```python
from build123d import *

# Parameters (mm, degrees)
F1_DEPTH = 10
F2_W     = 79.171128571
F2_H     = 17.1256698668
F3_DEPTH = 3
F6_R     = 24.75004298
F6_R_2   = 14.8028536267
F7_DEPTH = 3


# Not quite as in the source:
# - a fillet or chamfer that OpenCascade refuses, or shapes differently, is made with other operations: its cross-section is extruded or revolved along the edge and cut away or added


with BuildPart() as f1:
    # F0 (on Top) → F1 (new body)
    with BuildSketch(Plane.XY):
        with BuildLine():
            Line((-29.7593586147, -18.6613375429), (-29.7593586147, -52.9211238027))
            Line((-29.7593586147, -52.9211238027), (29.7593586147, -52.9211238027))
            Line((29.7593586147, -52.9211238027), (29.7593586147, -18.6613375429))
            ThreePointArc((29.7593586147, -18.6613375429), (0, -35.1264137658), (-29.7593586147, -18.6613375429))
        make_face()
        with BuildLine():
            ThreePointArc((-29.7593586147, 18.6613375429), (-35.1264137658, 0), (-29.7593586147, -18.6613375429))
            Line((-29.7593586147, -18.6613375429), (-29.7593586147, 18.6613375429))
        make_face()
        with BuildLine():
            Line((-29.7593586147, 18.6613375429), (-29.7593586147, -18.6613375429))
            ThreePointArc((-29.7593586147, -18.6613375429), (0, -35.1264137658), (29.7593586147, -18.6613375429))
            Line((29.7593586147, -18.6613375429), (29.7593586147, 18.6613375429))
            ThreePointArc((29.7593586147, 18.6613375429), (0, 35.1264137658), (-29.7593586147, 18.6613375429))
        make_face()
        with BuildLine():
            Line((29.7593586147, 18.6613375429), (29.7593586147, -18.6613375429))
            ThreePointArc((29.7593586147, -18.6613375429), (33.7579952615, -9.7088979792), (35.1264137658, 0))
            ThreePointArc((35.1264137658, 0), (33.7579952615, 9.7088979792), (29.7593586147, 18.6613375429))
        make_face()
        with BuildLine():
            Line((-29.7593586147, 52.9211238027), (-29.7593586147, 18.6613375429))
            ThreePointArc((-29.7593586147, 18.6613375429), (0, 35.1264137658), (29.7593586147, 18.6613375429))
            Line((29.7593586147, 18.6613375429), (29.7593586147, 52.9211238027))
            Line((29.7593586147, 52.9211238027), (-29.7593586147, 52.9211238027))
        make_face()
    extrude(amount=F1_DEPTH)

    # F2 (on Top) → F3 (cut)
    with BuildSketch(Plane.XY):
        Rectangle(F2_W, F2_H)
    extrude(amount=F3_DEPTH, mode=Mode.SUBTRACT)

    # F4 (on Front) → F5 (revolve, cut)
    with BuildSketch(Plane.XZ):
        with BuildLine():
            Line((0, -17.8640554044), (0, 17.8640554044))
            ThreePointArc((0, 17.8640554044), (-17.8640554044, 0), (0, -17.8640554044))
        make_face()
    revolve(axis=Axis((0, 0, 2.6136357337), (0, 0, 1)), mode=Mode.SUBTRACT)

    # F6 (on face) → F7 (join)
    with BuildSketch(Plane.XY.offset(10)):
        Circle(F6_R)
        Circle(F6_R_2, mode=Mode.SUBTRACT)
    extrude(amount=F7_DEPTH)

    # F8: fillet of radius 5 on 1 edges, made by hand

    # F8_s1 → F8_t2 (revolve, cut)
    with BuildSketch(Plane.XZ):
        with BuildLine():
            ThreePointArc((24.75004298, 10), (22.9060800725, 12.1833001327), (20.167467285, 13))
            Line((20.167467285, 13), (24.75004298, 13))
            Line((24.75004298, 13), (24.75004298, 10))
        make_face()
    revolve(axis=Axis((0, 0, 13), (0, 0, 1)), mode=Mode.SUBTRACT)


solid = f1.part
```
The model under review builds one solid part; all positions refer to its coordinate system, in mm. A direction names the side the tool comes from. Round coordinates to 2 decimals unless told otherwise and drop trailing zeros. Order: outer loops, then holes, each group sorted by start corner. A loop starts at its lowest first (then second) coordinate and runs counter-clockwise, first axis right, second up. Notation, with made-up numbers: (68.25, 31.25) -> (110.25, 31.25) arc R14 ccw to (110.25, 54.25) -> close; hole circle Ø7 at (-31.5, 68.25). An arc over 180 degrees is marked (long way). One line per item, written item: value. Start each with the question number.
Q1. Machinability: for faces 4 (the face through (25, -8.563, 1)), 5 (the face through (29.759, -36, 5)), 6 (the face through (7, 24, 10)), 7 (the face through (-29.759, 36, 5)), which of the approach directions +Z, -Z, +X, -X, +Y, -Y give a long, thin tool a straight path to every point of the face, cutting with its end or side? Answer none if there is none.
Q2. Wall thickness on line 1 (Z direction, x = -14.5, y = 37); line 2 (Y direction, x = 0, z = 11.05); line 3 (X direction, y = -7, z = 11.25): over which ranges is each line inside the solid? List them lowest first.
Q3. Take a section at B-B (z = 7). Write out the cut boundary in (x, y).
Q4. Take a section at A-A (x = 0). Write out the cut boundary in (y, z), and give its area (3 significant figures).
Q5. Take a section at C-C (y = -43.5). Write out the cut boundary in (x, z).
Q6. Clearance check with flat-ended pins moving along their axes: pin 1 Ø8.5 at (x, y) = (-23.5, 2.5) entering from -Z; pin 2 Ø5 at (y, z) = (33.5, 7.5) entering from -X; pin 3 Ø3 at (y, z) = (33.5, 4.5) entering from +X; pin 4 Ø8 at (x, y) = (27, -30) entering from -Z. State where each tip first meets the part, or that it passes through.
Q7. Mouldability with a two-part tool opening along Y and no side actions: class faces 1 (the face through (-35.125, 0.275, 6.041)), 2 (the face through (25, 8.563, 1)), 3 (the face through (-29.759, -36, 5)) as released by +Y, released by -Y, zero draft, split by the parting line, or undercut.
Reported:
1. face 4: -Z, +X, -X
1. face 5: +Z, -Z, +X, -Y
1. face 6: +Z
1. face 7: +Z, -Z, -X, +Y
2. line 1: z = 0 to 10
2. line 2: y = -24.13 to -14.8, 14.8 to 24.13
2. line 3: x = -22.92 to -13.04, 13.04 to 22.92
3. outline: (-29.76, -52.92) -> (29.76, -52.92) -> (29.76, -18.66) arc R35.13 ccw to (29.76, 18.66) -> (29.76, 52.92) -> (-29.76, 52.92) -> (-29.76, 18.66) arc R35.13 ccw to (-29.76, -18.66) -> close; hole circle Ø32.87 at (0, 0)
4. outline: (-52.92, 0) -> (-17.86, 0) arc R17.86 cw to (-14.8, 10) -> (-14.8, 13) -> (-20.17, 13) arc R5 ccw to (-24.75, 10) -> (-52.92, 10) -> close; (14.8, 10) arc R17.86 cw to (17.86, 0) -> (52.92, 0) -> (52.92, 10) -> (24.75, 10) arc R5 ccw to (20.17, 13) -> (14.8, 13) -> close
4. area: 773 mm2
5. outline: (-29.76, 0) -> (29.76, 0) -> (29.76, 10) -> (-29.76, 10) -> close
6. pin 1: stops at z = 3
6. pin 2: stops at x = -29.76
6. pin 3: stops at x = 29.76
6. pin 4: stops at z = 0
7. face 1: split by the parting line
7. face 2: undercut
7. face 3: zero draft
